Part model, mm, in its own coordinate system. A direction names the side the tool comes from. Round coordinates to 2 decimals unless told otherwise and drop trailing zeros. Write each loop counter-clockwise with the first axis right and the second up, starting at its lowest first coordinate (ties: lowest second). Pieces come first, ordered by that corner, then holes. Notation, with made-up numbers: M 9,49.25 L 27,49.25 A28 ccw 27,80.25 Z; hole C -19.5,51.5 d10. An arc over 180 degrees is marked long. One line per question, with ' | ' between items. Start each with the question number.
1) Saw through at D-D (x = 259). List the corners of the cut face in (y, z).
2) Saw through at C-C (z = -28.5). List the corners of the cut face in (x, y), plus the area to 3 significant figures.
3) Mould opens along X. For faces 5 (the face through (341.894, 3.605, -54.278)), 6 (the face through (447, 11, 127)), 7 (the face through (390.9, 0.17, 18.64)) say: pulls with the +X half, pulls with the -X half, needs draft (parallel to the pull), parting line crosses it, or undercut.
4) Saw through at A-A (y = 5.25). List the corners of the cut face in (x, z), plus the area to 3 significant figures.
5) Tool access for faces 1 (the face through (304.924, 0.168, 16.426)), 2 (the face through (376.04, -1.52, -13.77)), 3 (the face through (246.962, 3.605, 127.819)), 4 (the face through (432.047, 0.493, 107.915)): list every direction of +Z, -Z, +X, -X, +Y, -Y with a clear straight run to the whole face (end or side of a thin tool).
6) Wall check: probe 1 along Y at (x, z) = (360, -31); probe 2 along Z at (x, y) = (355, 3); probe 3 along X at (y, z) = (-0.5, 123.5). Give the ranges that are in metal, low to high. Write a range as [from, to].
7) Saw through at B-B (x = 369.5). List the corners of the cut face in (y, z), plus the area to 3 significant figures.
8) Drop flat-ended pins along their axis: pin 1 Ø1.8 at (x, z) = (392.5, 100.5) entering from +Y; pin 2 Ø1 at (y, z) = (-0.5, 126.5) entering from -X; pin 3 Ø3 at (y, z) = (-1.5, -44) entering from +X. Give the stop position or say it passes through.
```python
from build123d import *

# Parameters (mm, degrees)
SKETCH1_W                = 34.714871787
SKETCH1_H                = 10.923666426
BOSS_EXTRUDE1_DEPTH      = 1
BOSS_EXTRUDE2_DEPTH      = 11
BOSS_EXTRUDE3_DEPTH      = 5
BOSS_EXTRUDE3_DEPTH_BACK = 3
SKETCH3_W                = 50
SKETCH3_H                = 7
CUT_EXTRUDE3_DEPTH       = 25
SKETCH5_W                = 50
SKETCH5_H                = 7
CUT_EXTRUDE4_DEPTH       = 25
SKETCH6_W                = 50
SKETCH6_H                = 7
CUT_EXTRUDE5_DEPTH       = 25
SKETCH8_R                = 1.5
BOSS_EXTRUDE5_DEPTH      = 1
BOSS_EXTRUDE10_DEPTH     = 3


with BuildPart() as part:
    # Sketch1 → Boss-Extrude1 (new body)
    with BuildSketch(Plane(origin=(0, 0, 0), x_dir=(1, 0, 0), z_dir=(0, 1, 0))):
        Polygon((243.304219775, -116.484791865), (254.809280577, -136.408896137), (442.602090749, -136.409305398), (444.621046679, -132.925433224), (441.749040748, -132.925433224), (449.516726724, -119.471406458), (450.964695298, -121.978953123), (452.699916622, -118.984688018), (358.778179036, 43.666038065), (335.767496284, 43.666038065), align=None)
        with Locations((422.370878913, -129.522754792)):
            Rectangle(SKETCH1_W, SKETCH1_H, mode=Mode.SUBTRACT)
        Polygon((423.190377512, -92.577472767), (432.651287025, -87.114324326), (450.119365975, -117.364996826), (440.658456462, -122.828145267), align=None, mode=Mode.SUBTRACT)
        Polygon((428.113670919, -116.417164681), (266.439108268, -116.428009237), (347.273609729, 23.609230821), align=None, mode=Mode.SUBTRACT)
    extrude(amount=BOSS_EXTRUDE1_DEPTH)

    # Sketch1<9> → Boss-Extrude2 (add)
    # profile 1 of 2: a face of its own
    with BuildSketch(Plane(origin=(0, 0, 0), x_dir=(1, 0, 0), z_dir=(0, 1, 0))):
        Polygon((229.159432548, -134.984249184), (231.716666588, -139.412373829), (462.829865412, -139.412373829), (465.38624875, -134.984588004), (349.829542096, 65.165499075), (344.716133219, 65.165499075), align=None)
        Polygon((251.922647989, -136.409305399), (233.446303401, -136.408896138), (232.62355396, -134.984217357), (241.860901689, -118.984688018), align=None, mode=Mode.SUBTRACT)
        Polygon((442.602090749, -136.409305398), (254.809280577, -136.408896137), (243.304219775, -116.484791865), (335.767496284, 43.666038065), (358.778179036, 43.666038065), (461.938967958, -134.984588006), (461.116393749, -136.409305398), align=None, mode=Mode.SUBTRACT)
        Polygon((348.096628302, 62.164013367), (357.334800991, 46.166038067), (337.210874326, 46.166038067), (346.44844193, 62.165948237), align=None, mode=Mode.SUBTRACT)
    # profile 2 of 2: a face of its own
    with BuildSketch(Plane(origin=(0, 0, 0), x_dir=(1, 0, 0), z_dir=(0, 1, 0))):
        Polygon((441.749040748, -132.925433224), (444.621046679, -132.925433224), (450.964695298, -121.978953123), (449.516726724, -119.471406458), align=None)
    extrude(amount=BOSS_EXTRUDE2_DEPTH)

    # Sketch1<10> → Boss-Extrude3 (add, two sides: drawn at the far end of the back side and taken through both)
    # profile 1 of 2: a face of its own
    with BuildSketch(Plane(origin=(0, 0, 0), x_dir=(1, 0, 0), z_dir=(0, 1, 0)).offset(-BOSS_EXTRUDE3_DEPTH_BACK)):
        Polygon((229.159432548, -134.984249184), (231.716666588, -139.412373829), (462.829865412, -139.412373829), (465.38624875, -134.984588004), (349.829542096, 65.165499075), (344.716133219, 65.165499075), align=None)
        Polygon((251.922647989, -136.409305399), (233.446303401, -136.408896138), (232.62355396, -134.984217357), (241.860901689, -118.984688018), align=None, mode=Mode.SUBTRACT)
        Polygon((442.602090749, -136.409305398), (254.809280577, -136.408896137), (243.304219775, -116.484791865), (335.767496284, 43.666038065), (358.778179036, 43.666038065), (461.938967958, -134.984588006), (461.116393749, -136.409305398), align=None, mode=Mode.SUBTRACT)
        Polygon((348.096628302, 62.164013367), (357.334800991, 46.166038067), (337.210874326, 46.166038067), (346.44844193, 62.165948237), align=None, mode=Mode.SUBTRACT)
    # profile 2 of 2: a face of its own
    with BuildSketch(Plane(origin=(0, 0, 0), x_dir=(1, 0, 0), z_dir=(0, 1, 0)).offset(-BOSS_EXTRUDE3_DEPTH_BACK)):
        Polygon((441.749040748, -132.925433224), (444.621046679, -132.925433224), (450.964695298, -121.978953123), (449.516726724, -119.471406458), align=None)
    extrude(amount=BOSS_EXTRUDE3_DEPTH + BOSS_EXTRUDE3_DEPTH_BACK)

    # Sketch3 → Cut-Extrude3 (cut)
    with BuildSketch(Plane(origin=(290.589645397, 0, -167.772009994), x_dir=(-0.49999999999998745, 0, -0.8660254037844459), z_dir=(0.8660254037844459, 0, -0.49999999999998745))):
        with Locations((-236.592990632, -3)):
            Rectangle(SKETCH3_W, SKETCH3_H)
    extrude(amount=-CUT_EXTRUDE3_DEPTH, mode=Mode.SUBTRACT)

    # Sketch5 → Cut-Extrude4 (cut)
    with BuildSketch(Plane.XY.offset(139.412373829)):
        with Locations((347.273266, -3)):
            Rectangle(SKETCH5_W, SKETCH5_H)
    extrude(amount=-CUT_EXTRUDE4_DEPTH, mode=Mode.SUBTRACT)

    # Sketch6 → Cut-Extrude5 (cut)
    with BuildSketch(Plane(origin=(230.319375798, 0, 132.975171837), x_dir=(-0.5000006154012504, 0, 0.8660250484820695), z_dir=(-0.8660250484820695, 0, -0.5000006154012504))):
        with Locations((-113.236674799, -3)):
            Rectangle(SKETCH6_W, SKETCH6_H)
    extrude(amount=-CUT_EXTRUDE5_DEPTH, mode=Mode.SUBTRACT)

    # Sketch8 → Boss-Extrude5 (add)
    with BuildSketch(Plane.XZ.offset(3)):
        Polygon((349.829542096, -65.165499075), (465.38624875, 134.984588004), (462.829865412, 139.412373829), (231.716666588, 139.412373829), (229.159432548, 134.984249184), (344.716133219, -65.165499075), align=None)
        with Locations(Location((395.323540807, 98.692824234, 0), (0, 0, 270))):
            Circle(SKETCH8_R, mode=Mode.SUBTRACT)
        with Locations(Location((348.301285091, 15.863526629, 0), (0, 0, 270))):
            Circle(SKETCH8_R, mode=Mode.SUBTRACT)
        with Locations(Location((299.654911442, 97.24168178, 0), (0, 0, 270))):
            Circle(SKETCH8_R, mode=Mode.SUBTRACT)
        Polygon((444.621046679, 132.925433224), (450.964695298, 121.978953123), (449.516726724, 119.471406458), (427.347592194, 115.090208207), (404.33298615, 103.060878104), (405.774939109, 100.430142149), (424.549299543, 110.243170393), (451.871255231, 117.549638152), (452.699916622, 118.984688018), (461.938967958, 134.984588006), (461.116393749, 136.409305398), (442.602090749, 136.409305398), (439.019602541, 136.409297591), (420.379437571, 116.417683466), (402.410382205, 106.568526044), (403.852335164, 103.937790089), (426.620208946, 116.417264857), (441.749040748, 132.925433224), align=None, mode=Mode.SUBTRACT)
        Polygon((322.273266, 116.42426408), (294.358218631, 68.061097964), (319.354499367, 24.757680453), (376.473657316, 26.969372806), (401.47267951, 70.271207531), (372.273266, 116.420910257), align=None, mode=Mode.SUBTRACT)
        Polygon((233.446303401, 136.408896138), (251.922647989, 136.409305399), (241.860901689, 118.984688018), (232.62355396, 134.984217357), align=None, mode=Mode.SUBTRACT)
        Polygon((337.210874326, -46.166038067), (357.334800991, -46.166038067), (348.096628302, -62.164013367), (346.44844193, -62.165948237), align=None, mode=Mode.SUBTRACT)
    extrude(amount=BOSS_EXTRUDE5_DEPTH)

    # Sketch12 → Boss-Extrude10 (add)
    with BuildSketch(Plane(origin=(0, -3, 0), x_dir=(1, 0, 0), z_dir=(0, 1, 0))):
        with BuildLine():
            Line((347.417900211, -11.962292061), (347.307477101, -11.47463774))
            ThreePointArc((347.307477101, -11.47463774), (345.119304576, -12.681546114), (343.912396202, -14.869718639))
            Line((343.912396203, -14.869718639), (344.400050524, -14.980141749))
            ThreePointArc((344.400050523, -14.980141749), (345.472857967, -13.035099504), (347.417900211, -11.962292061))
        make_face()
        with BuildLine():
            ThreePointArc((352.690173981, -14.869718639), (351.483265607, -12.681546114), (349.295093082, -11.47463774))
            Line((349.295093081, -11.47463774), (349.184669971, -11.962292061))
            ThreePointArc((349.184669972, -11.962292061), (351.129712216, -13.035099504), (352.20251966, -14.980141749))
            Line((352.202519659, -14.980141749), (352.69017398, -14.869718639))
        make_face()
        with BuildLine():
            ThreePointArc((349.295093082, -20.252415518), (351.483265607, -19.045507145), (352.690173981, -16.857334619))
            Line((352.69017398, -16.857334619), (352.202519659, -16.746911509))
            ThreePointArc((352.20251966, -16.746911509), (351.129712216, -18.691953754), (349.184669972, -19.764761197))
            Line((349.184669971, -19.764761197), (349.295093081, -20.252415518))
        make_face()
        with BuildLine():
            Line((344.400050524, -16.746911509), (343.912396203, -16.857334619))
            ThreePointArc((343.912396202, -16.857334619), (345.119304576, -19.045507145), (347.307477101, -20.252415518))
            Line((347.307477101, -20.252415518), (347.417900211, -19.764761197))
            ThreePointArc((347.417900211, -19.764761197), (345.472857967, -18.691953754), (344.400050523, -16.746911509))
        make_face()
        with BuildLine():
            Line((394.440155927, -94.791589666), (394.329732817, -94.303935345))
            ThreePointArc((394.329732817, -94.303935345), (392.141560292, -95.510843718), (390.934651918, -97.699016244))
            Line((390.934651918, -97.699016244), (391.4247896, -97.798542945))
            ThreePointArc((391.4247896, -97.798542945), (392.499067689, -95.860448622), (394.440155927, -94.791589666))
        make_face()
        with BuildLine():
            ThreePointArc((399.712429696, -97.699016244), (398.505521323, -95.510843718), (396.317348797, -94.303935345))
            Line((396.317348797, -94.303935345), (396.206925687, -94.791589666))
            ThreePointArc((396.206925687, -94.791589666), (398.151967932, -95.864397109), (399.224775375, -97.809439354))
            Line((399.224775375, -97.809439354), (399.712429696, -97.699016244))
        make_face()
        with BuildLine():
            ThreePointArc((396.317348797, -103.081713123), (398.505521323, -101.874804749), (399.712429696, -99.686632224))
            Line((399.712429696, -99.686632224), (399.224775375, -99.576209114))
            ThreePointArc((399.224775375, -99.576209114), (398.151967932, -101.521251358), (396.206925687, -102.594058802))
            Line((396.206925687, -102.594058801), (396.317348797, -103.081713122))
        make_face()
        with BuildLine():
            Line((391.422306239, -99.576209114), (390.934651918, -99.686632224))
            ThreePointArc((390.934651918, -99.686632224), (392.141560292, -101.874804749), (394.329732817, -103.081713123))
            Line((394.329732817, -103.081713122), (394.440155927, -102.594058801))
            ThreePointArc((394.440155927, -102.594058802), (392.495113682, -101.521251358), (391.422306239, -99.576209114))
        make_face()
        with BuildLine():
            ThreePointArc((298.661103452, -92.852792892), (296.472930927, -94.059701265), (295.266022553, -96.24787379))
            Line((295.266022553, -96.24787379), (295.753676874, -96.3582969))
            ThreePointArc((295.753676874, -96.3582969), (296.826484317, -94.413254656), (298.771526562, -93.340447213))
            Line((298.771526562, -93.340447212), (298.661103452, -92.852792891))
        make_face()
        with BuildLine():
            ThreePointArc((304.04380033, -96.24787379), (302.836891957, -94.059701265), (300.648719432, -92.852792892))
            Line((300.648719432, -92.852792891), (300.538296322, -93.340447212))
            ThreePointArc((300.538296322, -93.340447213), (302.483338566, -94.413254656), (303.55614601, -96.3582969))
            Line((303.55614601, -96.3582969), (304.043800331, -96.24787379))
        make_face()
        with BuildLine():
            Line((300.538296322, -101.142916348), (300.648719432, -101.630570669))
            ThreePointArc((300.648719432, -101.630570669), (302.836891957, -100.423662295), (304.04380033, -98.23548977))
            Line((304.043800331, -98.23548977), (303.55614601, -98.12506666))
            ThreePointArc((303.55614601, -98.12506666), (302.483338566, -100.070108905), (300.538296322, -101.142916348))
        make_face()
        with BuildLine():
            Line((295.753676874, -98.12506666), (295.266022553, -98.23548977))
            ThreePointArc((295.266022553, -98.23548977), (296.472930927, -100.423662295), (298.661103452, -101.630570669))
            Line((298.661103452, -101.630570669), (298.771526562, -101.142916348))
            ThreePointArc((298.771526562, -101.142916348), (296.826484317, -100.070108905), (295.753676874, -98.12506666))
        make_face()
    extrude(amount=BOSS_EXTRUDE10_DEPTH)


solid = part.part
```
Answer key:
1) outline: M -4,83.3 L 11,83.3 L 11,89.3 L 1,89.3 L 1,136.41 L 11,136.41 L 11,139.41 L -4,139.41 Z; hole M -3,89.3 L 0,89.3 L 0,136.41 L -3,136.41 Z
2) outline: M 323.55,-4 L 371,-4 L 371,11 L 367.54,11 L 367.54,1 L 327.01,1 L 327.01,11 L 323.55,11 Z; hole M 327.01,-3 L 367.54,-3 L 367.54,0 L 327.01,0 Z | area: 185 mm2
3) face 5: undercut | face 6: needs draft | face 7: pulls with the +X half
4) outline: M 229.16,134.98 L 344.72,-65.17 L 349.83,-65.17 L 465.39,134.98 L 462.83,139.41 L 231.72,139.41 Z; M 441.75,132.93 L 449.52,119.47 L 450.96,121.98 L 444.62,132.93 Z; hole M 232.62,134.98 L 241.86,118.98 L 251.92,136.41 L 233.45,136.41 Z; hole M 243.3,116.48 L 335.77,-43.67 L 358.78,-43.67 L 461.94,134.98 L 461.12,136.41 L 442.6,136.41 L 254.81,136.41 Z; hole M 337.21,-46.17 L 346.45,-62.17 L 348.1,-62.16 L 357.33,-46.17 Z | area: 2,240 mm2
5) face 1: -X | face 2: none | face 3: +Y, -Y | face 4: +Y
6) probe 1: y = [-4, -3], [0, 1] | probe 2: z = [-56.21, -50.21], [-46.17, -43.67], [136.41, 139.41] | probe 3: x = [235.79, 239.25], [244.47, 247.36], [447.19, 450.08], [455.31, 458.76]
7) outline: M -4,-31.1 L 11,-31.1 L 11,-25.1 L 1,-25.1 L 1,14.89 L 0,14.89 L 0,-25.1 L -3,-25.1 L -3,26.7 L -4,26.7 Z; M -4,116.42 L -3,116.42 L -3,139.41 L -4,139.41 Z; M 0.5,116.42 L 1,116.42 L 1,136.41 L 11,136.41 L 11,139.41 L 0.5,139.41 Z | area: 246 mm2
8) pin 1: stops at y = 0 | pin 2: stops at x = 233.77 | pin 3: stops at x = 362.92
